from build123d import *

# Parameters (mm, degrees)
SKETCH_1_R          = 1.5
EXTRUDE_2_DEPTH     = 5
CUT_EXTRUDE_1_DEPTH = 1
SKETCH_5_W          = 20
SKETCH_5_H          = 40
EXTRUDE_3_DEPTH     = 3
SKETCH_6_R          = 1.55
CUT_EXTRUDE_2_DEPTH = 10


with BuildPart() as part:
    # 草图1 → 凸台-拉伸2 (new body)
    with BuildSketch(Plane(origin=(0, 0, 0), x_dir=(0, 0, -1), z_dir=(1, 0, 0))):
        with BuildLine():
            Line((-15, 0), (15, 0))
            Line((15, 0), (15, 130))
            ThreePointArc((15, 130), (16.060667235, 133.763397528), (17.833287426, 137.248507798))
            Line((17.833287426, 137.248507798), (34.277601095, 169.80605943))
            ThreePointArc((34.277601095, 169.80605943), (22.969406924, 178.256928012), (10.37531975, 171.878730504))
            Line((10.37531975, 171.878730504), (-12.166712574, 127.248507798))
            ThreePointArc((-12.166712574, 127.248507798), (-13.939332765, 123.763397528), (-15, 120))
            Line((-15, 120), (-15, 0))
        make_face()
        with Locations((0, 23.934052351)):
            Circle(SKETCH_1_R, mode=Mode.SUBTRACT)
        with Locations((0, 47.934052351)):
            Circle(SKETCH_1_R, mode=Mode.SUBTRACT)
        with Locations((0, 71.934052351)):
            Circle(SKETCH_1_R, mode=Mode.SUBTRACT)
        with Locations((0, 95.934052351)):
            Circle(SKETCH_1_R, mode=Mode.SUBTRACT)
        with Locations((10.541707006, 142.602806473)):
            Circle(SKETCH_1_R, mode=Mode.SUBTRACT)
        with Locations((0, 119.934052351)):
            Circle(SKETCH_1_R, mode=Mode.SUBTRACT)
        with Locations((21.812723168, 164.917917825)):
            Circle(SKETCH_1_R, mode=Mode.SUBTRACT)
        with Locations((11.964645637, 166.654399602)):
            Circle(SKETCH_1_R, mode=Mode.SUBTRACT)
        with Locations((11.964645637, 163.181436049)):
            Circle(SKETCH_1_R, mode=Mode.SUBTRACT)
        with Locations((13.15246913, 159.917917825)):
            Circle(SKETCH_1_R, mode=Mode.SUBTRACT)
        with Locations((15.384847071, 157.257473394)):
            Circle(SKETCH_1_R, mode=Mode.SUBTRACT)
        with Locations((18.392521734, 155.520991617)):
            Circle(SKETCH_1_R, mode=Mode.SUBTRACT)
        with Locations((21.812723168, 154.917917825)):
            Circle(SKETCH_1_R, mode=Mode.SUBTRACT)
        with Locations((13.15246913, 169.917917825)):
            Circle(SKETCH_1_R, mode=Mode.SUBTRACT)
        with Locations((15.384847071, 172.578362256)):
            Circle(SKETCH_1_R, mode=Mode.SUBTRACT)
        with Locations((18.392521734, 174.314844033)):
            Circle(SKETCH_1_R, mode=Mode.SUBTRACT)
        with Locations((21.812723168, 174.917917825)):
            Circle(SKETCH_1_R, mode=Mode.SUBTRACT)
    extrude(amount=-EXTRUDE_2_DEPTH)

    # 草图4 → 切除-拉伸1 (cut)
    with BuildSketch(Plane(origin=(0, 0, 0), x_dir=(0, 0, -1), z_dir=(1, 0, 0))):
        with BuildLine():
            Line((-10, 5), (10, 5))
            Line((10, 5), (10, 130.418298195))
            ThreePointArc((10, 130.418298195), (11.272736422, 135.241025308), (13.477541954, 139.715104809))
            Line((13.477541954, 139.715104809), (28.657153069, 169.768713769))
            ThreePointArc((28.657153069, 169.768713769), (21.607154469, 173.304465594), (14.73885303, 169.427552317))
            Line((14.73885303, 169.427552317), (-7.82549521, 124.753147068))
            ThreePointArc((-7.82549521, 124.753147068), (-9.161705076, 122.242477333), (-10, 119.524724411))
            Line((-10, 119.524724411), (-10, 5))
        make_face()
    extrude(amount=-CUT_EXTRUDE_1_DEPTH, mode=Mode.SUBTRACT)

    # 草图5 → 凸台-拉伸3 (add)
    with BuildSketch(Plane(origin=(0, 0, 0), x_dir=(-1, 0, 0), z_dir=(0, -1, 0))):
        with Locations((10, 5)):
            Rectangle(SKETCH_5_W, SKETCH_5_H)
    extrude(amount=-EXTRUDE_3_DEPTH)

    # 草图6 → 切除-拉伸2 (cut)
    with BuildSketch(Plane.XZ):
        with Locations(Location((-13, -18, 0), (0, 0, 270))):
            Circle(SKETCH_6_R)
        with Locations(Location((-13, 8, 0), (0, 0, 270))):
            Circle(SKETCH_6_R)
    extrude(amount=-CUT_EXTRUDE_2_DEPTH, mode=Mode.SUBTRACT)


solid = part.part
The model under review builds one solid part; all positions refer to its coordinate system, in mm. A direction names the side the tool comes from. Coordinates: 2 decimals unless noted, no trailing zeros. Write each loop counter-clockwise with the first axis right and the second up, starting at its lowest first coordinate (ties: lowest second). Pieces come first, ordered by that corner, then holes. Notation, with made-up numbers: (23.25, 45) - (81.25, 45) arc R8 ccw to (81.25, 56) - close; hole circle Ø8 at (39.5, -32.5). An arc over 180 degrees is marked (long way). Answer as a JSON object with one key per item and string values. Group by question number.
1. Add section A-A (x = -13). Give the boundary of the cut face in (y, z), plus the area to 3 significant figures.
2. Clearance check with flat-ended pins moving along their axes: pin 1 Ø4 at (y, z) = (156, -11.5) entering from -X; pin 2 Ø0.5 at (x, y) = (-0.5, 84.5) entering from -Z; pin 3 Ø0.8 at (x, z) = (-0.5, 0.5) entering from +Y; pin 4 Ø1.5 at (x, y) = (-7, 83) entering from +Z. State where each tip first meets the part, or that it passes through.
3. Mouldability with a two-part tool opening along Z and no side actions: class faces 4 (the face through (-2.972, 163.454, -21.488)), 5 (the face through (-2.46, 123.81, 13.92)), 6 (the face through (-0.49, 163, -25.24)), 7 (the face through (-10, 0, -5)) as pulls with the +Z half, pulls with the -Z half, needs draft (parallel to the pull), parting line crosses it, or undercut.
4. To check wall thickness, follow probe 1 along X at (y, z) = (45, 1); probe 2 along Y at (x, z) = (-16.5, 11); probe 3 along Y at (x, z) = (-2.95, 0). State the ranges of each line that lie inside material, in increasing order.
5. Add section B-B (y = 51). Give the boundary of the cut face in (x, z), plus the area to 3 significant figures.
6. Add section C-C (z = 0). Give the number of separate pieces and of enclosed holes in the cut face, plus the area to 3 significant figures.
7. Machinability: for faces 1 (the face through (-2.465, 163.247, -10.466)), 2 (the face through (-0.49, 135.18, -11.25)), 3 (the face through (-2, 66, -15)), which of the approach directions +Z, -Z, +X, -X, +Y, -Y give a long, thin tool a straight path to every point of the face, cutting with its end or side? Answer none if there is none.
Findings:
{
 "1": {"outline": "(0, -25) - (3, -25) - (3, -19.55) - (0, -19.55) - close; (0, -16.45) - (3, -16.45) - (3, 6.45) - (0, 6.45) - close; (0, 9.55) - (3, 9.55) - (3, 15) - (0, 15) - close", "area": "101 mm²"},
 "2": {"pin 1": "x = -5", "pin 2": "z = -15", "pin 3": "y = 151.14", "pin 4": "through"},
 "3": {"face 4": "undercut", "face 5": "pulls with the +Z half", "face 6": "undercut", "face 7": "needs draft"},
 "4": {"probe 1": "-5 to -1", "probe 2": "0 to 3", "probe 3": "0 to 22.43, 25.43 to 46.43, 49.43 to 70.43, 73.43 to 94.43, 97.43 to 118.43, 121.43 to 151.34"},
 "5": {"outline": "(-5, -15) - (0, -15) - (0, -10) - (-1, -10) - (-1, 10) - (0, 10) - (0, 15) - (-5, 15) - close", "area": "130 mm²"},
 "6": {"separate pieces": "6", "enclosed holes": "0", "area": "606 mm²"},
 "7": {"face 1": "+X, -X", "face 2": "+X", "face 3": "-Z, +X, -X"}
}
